from build123d import *

# Parameters (mm, degrees)
BOSS_EXTRUDE1_DEPTH = 6.35
SKETCH2_R           = 9.525
BOSS_EXTRUDE2_DEPTH = 101.6
FILLET1_R           = 1.27
SKETCH3_R           = 5.08
CUT_EXTRUDE1_DEPTH  = 8.89
CHAMFER1_SIZE       = 1.27
SKETCH9_R           = 0.9525
CUT_EXTRUDE2_DEPTH  = 130.310350126
SKETCH10_R          = 2.54
CUT_EXTRUDE3_DEPTH  = 130.310350126
CHAMFER2_SIZE       = 1.27
SKETCH11_R          = 1.524
CUT_EXTRUDE4_DEPTH  = 135.357021215
SKETCH12_R          = 1.89865
CUT_EXTRUDE5_DEPTH  = 130.310350126


with BuildPart() as part:
    # Sketch1 → Boss-Extrude1 (new body)
    with BuildSketch(Plane(origin=(0, 0, 0), x_dir=(1, 0, 0), z_dir=(0, 1, 0))):
        Polygon((18.605162135, -55.630039325), (57.479608336, -11.702476612), (38.874446201, 43.927562713), (-18.605162135, 55.630039325), (-57.479608336, 11.702476612), (-38.874446201, -43.927562713), align=None)
    extrude(amount=BOSS_EXTRUDE1_DEPTH)

    # Sketch2 → Boss-Extrude2 (add)
    with BuildSketch(Plane(origin=(0, 6.35, 0), x_dir=(1, 0, 0), z_dir=(0, 1, 0))):
        with Locations(Location((0, 0, 0), (0, 0, 270))):
            Circle(SKETCH2_R)
    extrude(amount=BOSS_EXTRUDE2_DEPTH)

    # Fillet1
    fillet1_edges = [part.edges().sort_by_distance(p)[0] for p in [
        (0, 6.35, -9.525),
    ]]
    fillet(fillet1_edges, radius=FILLET1_R)

    # Sketch3 → Cut-Extrude1 (cut)
    with BuildSketch(Plane(origin=(0, 107.95, 0), x_dir=(1, 0, 0), z_dir=(0, 1, 0))):
        with Locations(Location((0, 0, 0), (0, 0, 270))):
            Circle(SKETCH3_R)
    extrude(amount=-CUT_EXTRUDE1_DEPTH, mode=Mode.SUBTRACT)

    # Chamfer1
    chamfer1_edges = [part.edges().sort_by_distance(p)[0] for p in [
        (0, 107.95, -5.08),
    ]]
    chamfer(chamfer1_edges, length=CHAMFER1_SIZE)

    # Sketch9 → Cut-Extrude2 (cut, through all)
    with BuildSketch(Plane(origin=(0, 6.35, 0), x_dir=(1, 0, 0), z_dir=(0, 1, 0))):
        with Locations(Location((-5.682110904, -12.762230043, 0), (0, 0, 270))):
            Circle(SKETCH9_R)
    extrude(amount=-CUT_EXTRUDE2_DEPTH, mode=Mode.SUBTRACT)

    # Sketch10 → Cut-Extrude3 (cut, through all)
    with BuildSketch(Plane(origin=(0, 6.35, 0), x_dir=(1, 0, 0), z_dir=(0, 1, 0))):
        with Locations(Location((-25.854998031, 0, 0), (0, 0, 270))):
            Circle(SKETCH10_R)
        with Locations(Location((25.854998031, 0, 0), (0, 0, 270))):
            Circle(SKETCH10_R)
    extrude(amount=-CUT_EXTRUDE3_DEPTH, mode=Mode.SUBTRACT)

    # Chamfer2
    chamfer2_edges = [part.edges().sort_by_distance(p)[0] for p in [
        (-25.854998031, 6.35, -2.54),
        (25.854998031, 6.35, -2.54),
    ]]
    chamfer(chamfer2_edges, length=CHAMFER2_SIZE)

    # Sketch11 → Cut-Extrude4 (cut, through all)
    with BuildSketch(Plane.XZ):
        with Locations(Location((11.278780135, 33.723919088, 0), (0, 0, 270))):
            Circle(SKETCH11_R)
        with Locations(Location((34.845160713, 7.094249423, 0), (0, 0, 270))):
            Circle(SKETCH11_R)
        with Locations(Location((23.566380578, -26.629669665, 0), (0, 0, 270))):
            Circle(SKETCH11_R)
        with Locations(Location((-11.278780135, -33.723919088, 0), (0, 0, 270))):
            Circle(SKETCH11_R)
        with Locations(Location((-34.845160713, -7.094249423, 0), (0, 0, 270))):
            Circle(SKETCH11_R)
        with Locations(Location((-23.566380578, 26.629669665, 0), (0, 0, 270))):
            Circle(SKETCH11_R)
    extrude(amount=-CUT_EXTRUDE4_DEPTH, mode=Mode.SUBTRACT)

    # Sketch12 → Cut-Extrude5 (cut, through all)
    with BuildSketch(Plane(origin=(0, 6.35, 0), x_dir=(1, 0, 0), z_dir=(0, 1, 0))):
        with Locations(Location((-47.589870854, -0.850796432, 0), (0, 0, 270))):
            Circle(SKETCH12_R)
        with Locations(Location((-38.526565389, -27.95037427, 0), (0, 0, 270))):
            Circle(SKETCH12_R)
        with Locations(Location((-43.469016858, 19.389797212, 0), (0, 0, 270))):
            Circle(SKETCH12_R)
        with Locations(Location((-24.531746751, 40.788638907, 0), (0, 0, 270))):
            Circle(SKETCH12_R)
        with Locations(Location((-4.942451469, 47.340171482, 0), (0, 0, 270))):
            Circle(SKETCH12_R)
        with Locations(Location((23.058124104, 41.639435339, 0), (0, 0, 270))):
            Circle(SKETCH12_R)
        with Locations(Location((38.526565389, 27.95037427, 0), (0, 0, 270))):
            Circle(SKETCH12_R)
        with Locations(Location((47.589870854, 0.850796432, 0), (0, 0, 270))):
            Circle(SKETCH12_R)
        with Locations(Location((43.469016858, -19.389797212, 0), (0, 0, 270))):
            Circle(SKETCH12_R)
        with Locations(Location((24.531746751, -40.788638907, 0), (0, 0, 270))):
            Circle(SKETCH12_R)
        with Locations(Location((4.942451469, -47.340171482, 0), (0, 0, 270))):
            Circle(SKETCH12_R)
        with Locations(Location((-23.058124104, -41.639435339, 0), (0, 0, 270))):
            Circle(SKETCH12_R)
    extrude(amount=-CUT_EXTRUDE5_DEPTH, mode=Mode.SUBTRACT)


solid = part.part
The model under review builds one solid part; all positions refer to its coordinate system, in mm. Round coordinates to 2 decimals unless told otherwise and drop trailing zeros. Loops run counter-clockwise (first coordinate to the right, second up) from the corner with the lowest first, then second, coordinate; pieces in that order, holes last. Notation, with made-up numbers: (14, -8) -> (26, -8) arc R23 cw to (26, 27) -> close; hole circle Ø5 at (42.25, -32). An arc over 180 degrees is marked (long way). Answer as CSV lines item,"result".
1) For P1, Ø5, axis at x = -2, z = 0, coming from the +Y side; P2, Ø5, axis at x = 4.94, z = 47.34, coming from the +Y side, all flat-tipped, find the tip position at first contact; note any pin that passes through.
Geometry results:
P1,"stops at y = 99.06"
P2,"stops at y = 6.35"
2) Add section A-A on x = 0. Write out the cut boundary in (y, z) (3 decimals).
Geometry results:
outline,"(0, -51.842) -> (6.35, -51.842) -> (6.35, -10.795) arc R1.27 cw to (7.62, -9.525) -> (107.95, -9.525) -> (107.95, -6.35) -> (106.68, -5.08) -> (99.06, -5.08) -> (99.06, 5.08) -> (106.68, 5.08) -> (107.95, 6.35) -> (107.95, 9.525) -> (7.62, 9.525) arc R1.27 cw to (6.35, 10.795) -> (6.35, 51.842) -> (0, 51.842) -> close"
3) Add section B-B on y = 61.5. Write out the cut boundary in (x, z) (3 decimals).
Geometry results:
outline,"circle Ø19.05 at (0, 0)"
4) Draft analysis for pull direction Z (two halves, no side actions). For faces 1 (the face through (-5.796, 57.083, -7.559)), 2 (the face through (0, 99.06, 0)), 3 (the face through (-10.537, 3.131, 49.697)), state which applies: pulls with the +Z half, pulls with the -Z half, needs draft (parallel to the pull), parting line crosses it, or undercut.
Geometry results:
face 1,"parting line crosses it"
face 2,"undercut"
face 3,"pulls with the +Z half"
5) To check wall thickness, follow line 1 along Y through (x, z) = (45, -5.5); line 2 along Z through (x, y) = (-4, 88.5); line 3 along X through (y, z) = (32, 7). State the ranges of each line that lie inside material, in increasing order. Write a range as from..to.
Geometry results:
line 1,"y = 0..6.35"
line 2,"z = -8.64..8.64"
line 3,"x = -6.46..6.46"
